Can you work these out from the model? Positions are in its coordinate system, mm. A direction names the side the tool comes from. Give positions to 0.01 mm unless a question says otherwise; leave off trailing zeros. Order: outer loops, then holes, each group sorted by start corner. A loop starts at its lowest first (then second) coordinate and runs counter-clockwise, first axis right, second up. Notation, with made-up numbers: (83.25, 19.5) - (98.25, 19.5) arc R15 ccw to (98.25, 39.5) - close; hole circle Ø11 at (81, -6.5). An arc over 180 degrees is marked (long way). Answer as CSV lines item,"result".
```python
from build123d import *

# Parameters (mm, degrees)
BASE_FLANGE1_DEPTH = 3.175
FILLET1_R          = 6.35
FILLET2_R          = 19.05
FILLET3_R          = 3.175
SKETCH3_R          = 4.396875001
CUT_EXTRUDE1_DEPTH = 3.175


# Sheet-metal steps are written as plain solids
with BuildPart() as part:
    # Sketch1 → Base-Flange1 (new body)
    with BuildSketch(Plane.XY):
        Polygon((0, 0), (41.397840965, 0), (41.397840965, 54.644007143), (19.045840965, 54.644007143), (19.045840965, 22.352), (0, 22.352), align=None)
    extrude(amount=-BASE_FLANGE1_DEPTH)

    # Fillet1
    fillet1_edges = [part.edges().sort_by_distance(p)[0] for p in [
        (0, 22.352, -1.5875),
        (19.045840965, 54.644007143, -1.5875),
        (41.397840965, 54.644007143, -1.5875),
        (0, 0, -1.5875),
    ]]
    fillet(fillet1_edges, radius=FILLET1_R)

    # Fillet2
    fillet2_edges = [part.edges().sort_by_distance(p)[0] for p in [
        (41.397840965, 0, -1.5875),
    ]]
    fillet(fillet2_edges, radius=FILLET2_R)

    # Fillet3
    fillet3_edges = [part.edges().sort_by_distance(p)[0] for p in [
        (19.045840965, 22.352, -1.5875),
    ]]
    fillet(fillet3_edges, radius=FILLET3_R)

    # Sketch3 → Cut-Extrude1 (cut)
    with BuildSketch(Plane.XY):
        with Locations((30.221840965, 45.119007143)):
            Circle(SKETCH3_R)
        with BuildLine():
            Line((10.93094867, 12.325), (10.93094867, 7.325))
            ThreePointArc((10.93094867, 7.325), (8.18094867, 4.575), (5.43094867, 7.325))
            Line((5.43094867, 7.325), (5.43094867, 12.325))
            ThreePointArc((5.43094867, 12.325), (8.18094867, 15.075), (10.93094867, 12.325))
        make_face()
    extrude(amount=-CUT_EXTRUDE1_DEPTH, mode=Mode.SUBTRACT)


solid = part.part
```
1) I want a section at B-B on z = -0.95. Write out the boundary of the cut face in (x, y) (3 decimals).
Answer block:
outline,"(0, 6.35) arc R6.35 ccw to (6.35, 0) - (22.348, 0) arc R19.05 ccw to (41.398, 19.05) - (41.398, 48.294) arc R6.35 ccw to (35.048, 54.644) - (25.396, 54.644) arc R6.35 ccw to (19.046, 48.294) - (19.046, 25.527) arc R3.175 cw to (15.871, 22.352) - (6.35, 22.352) arc R6.35 ccw to (0, 16.002) - close; hole (5.431, 7.325) arc R2.75 ccw to (10.931, 7.325) - (10.931, 12.325) arc R2.75 ccw to (5.431, 12.325) - close; hole circle Ø8.794 at (30.222, 45.119)"
2) I need wall thicknesses on line 1 along X through (y, z) = (25.5, -1.5); line 2 along Y through (x, z) = (10.5, -2.35); line 3 along Y through (x, z) = (6.5, -2.95). Which ranges of each line are inside material? Lowest first, please. Write a range as [from, to].
Answer block:
line 1,"[19.05, 41.4]"
line 2,"[0, 5.85], [13.8, 22.35]"
line 3,"[0, 5.15], [14.5, 22.35]"
3) I want a section at C-C on y = 41.5. Write out the boundary of the cut face in (x, z) (3 decimals).
Answer block:
outline,"(19.046, -3.175) - (27.725, -3.175) - (27.725, 0) - (19.046, 0) - close; (32.719, -3.175) - (41.398, -3.175) - (41.398, 0) - (32.719, 0) - close"
4) I'm going to push flat-ended pins straight in: P1, Ø1, axis at y = 27.5, z = -1.5, coming from the -X side; P2, Ø1, axis at x = 13, z = -2, coming from the +Y side; P3, Ø1.6, axis at y = 10, z = -2, coming from the +X side. Where does each tip first touch, or does it pass through?
Answer block:
P1,"x = 19.05"
P2,"y = 22.35"
P3,"x = 39.52"
5) Which directions (+Z, -Z, +X, -X, +Y, -Y) give clear straight access to the entire face, cutting with the end or side of a thin tool? Please do faces 4 (the flat face through (14, 0, -2)), 5 (the flat face through (10.931, 10, -2)), 6 (the flat face through (19.046, 37, -2)).
Answer block:
face 4,"+Z, -Z, +X, -X, -Y"
face 5,"+Z, -Z"
face 6,"+Z, -Z, -X, +Y"
6) I want a section at A-A on x = 29.5. Write out the boundary of the cut face in (y, z) (3 decimals), plus the area to 3 significant figures.
Answer block:
outline,"(1.394, -3.175) - (40.782, -3.175) - (40.782, 0) - (1.394, 0) - close; (49.456, -3.175) - (54.644, -3.175) - (54.644, 0) - (49.456, 0) - close"
area,"142 mm2"
7) If we mould it in two halves opening along X, with no side actions, what happens to faces 1 (the flat face through (5.431, 10, -2)), 2 (the cylindrical face through (35.669, 5.432, -1.61)), 3 (the flat face through (25, 22, -3.175))? For each: +X half, -X half, draft (parallel to the pull), parting line (faces both ways), or undercut.
Answer block:
face 1,"undercut"
face 2,"+X half"
face 3,"draft"
8) I want a section at D-D on x = 13.5. Write out the boundary of the cut face in (y, z) (3 decimals), plus the area to 3 significant figures.
Answer block:
outline,"(0, -3.175) - (22.352, -3.175) - (22.352, 0) - (0, 0) - close"
area,"71.0 mm2"
